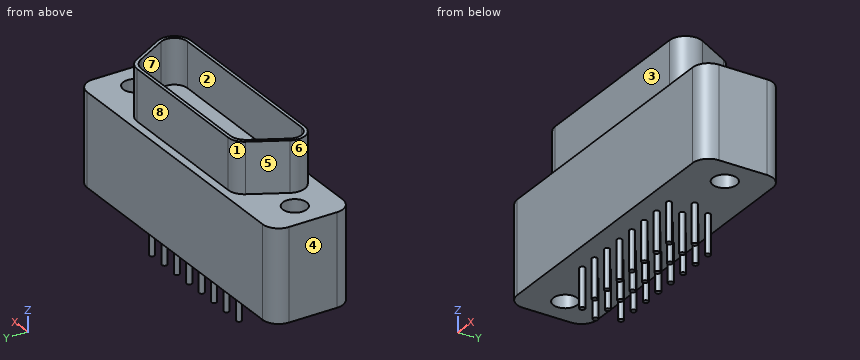
from build123d import *

# Parameters (mm, degrees)
F0_R     = 1.1684
F1_DEPTH = 4.5085
F3_DEPTH = 4.953
F5_DEPTH = 4.4069
F6_R     = 0.254
F7_DEPTH = 3.81


with BuildPart() as f1:
    # F0 (on Top) → F1 (new body, symmetric)
    with BuildSketch(Plane.XY):
        with BuildLine():
            Line((13.4747, 3.937), (-13.4747, 3.937))
            ThreePointArc((-13.4747, 3.937), (-14.588252, 3.475752), (-15.0495, 2.3622))
            Line((-15.0495, 2.3622), (-15.0495, -2.3622))
            ThreePointArc((-15.0495, -2.3622), (-14.588252, -3.475752), (-13.4747, -3.937))
            Line((-13.4747, -3.937), (13.4747, -3.937))
            ThreePointArc((13.4747, -3.937), (14.588252, -3.475752), (15.0495, -2.3622))
            Line((15.0495, -2.3622), (15.0495, 2.3622))
            ThreePointArc((15.0495, 2.3622), (14.588252, 3.475752), (13.4747, 3.937))
        make_face()
        with Locations((-12.2555, 0)):
            Circle(F0_R, mode=Mode.SUBTRACT)
        with Locations((12.2555, 0)):
            Circle(F0_R, mode=Mode.SUBTRACT)
    extrude(amount=F1_DEPTH, both=True)

    # F2 (on face) → F3 (join)
    with BuildSketch(Plane.XY.offset(4.5085)):
        with BuildLine():
            Line((-8.78192, -3.2004), (8.783378, -3.2004))
            ThreePointArc((8.783378, -3.2004), (10.140271, -2.424871), (10.160729, -0.862122))
            Line((10.160729, -0.862122), (8.372639, 2.363678))
            ThreePointArc((8.372639, 2.363678), (7.794559, 2.957094), (6.995288, 3.175))
            Line((6.995288, 3.175), (-6.99383, 3.175))
            ThreePointArc((-6.99383, 3.175), (-7.793101, 2.957094), (-8.371181, 2.363678))
            Line((-8.371181, 2.363678), (-10.159271, -0.862122))
            ThreePointArc((-10.159271, -0.862122), (-10.138814, -2.424871), (-8.78192, -3.2004))
        make_face()
    extrude(amount=F3_DEPTH)

    # F4 (on face) → F5 (cut)
    with BuildSketch(Plane.XY.offset(9.4615)):
        with BuildLine():
            Line((6.808266, 2.8575), (-6.806808, 2.8575))
            ThreePointArc((-6.806808, 2.8575), (-7.60608, 2.639594), (-8.184159, 2.046178))
            Line((-8.184159, 2.046178), (-9.871127, -0.997192))
            ThreePointArc((-9.871127, -0.997192), (-9.854629, -2.257474), (-8.76036, -2.8829))
            Line((-8.76036, -2.8829), (8.761817, -2.8829))
            ThreePointArc((8.761817, -2.8829), (9.856086, -2.257474), (9.872584, -0.997192))
            Line((9.872584, -0.997192), (8.185617, 2.046178))
            ThreePointArc((8.185617, 2.046178), (7.607537, 2.639594), (6.808266, 2.8575))
        make_face()
    extrude(amount=-F5_DEPTH, mode=Mode.SUBTRACT)

    # F6 (on face) → F7 (join)
    with BuildSketch(Plane(origin=(0, 0, -4.5085), x_dir=(1, 0, 0), z_dir=(0, 0, -1))):
        with Locations((-6.6548, 1.905)):
            Circle(F6_R)
        with Locations((-4.7498, 1.905)):
            Circle(F6_R)
        with Locations((-2.8448, 1.905)):
            Circle(F6_R)
        with Locations((-0.9398, 1.905)):
            Circle(F6_R)
        with Locations((0.9652, 1.905)):
            Circle(F6_R)
        with Locations((2.8702, 1.905)):
            Circle(F6_R)
        with Locations((4.7752, 1.905)):
            Circle(F6_R)
        with Locations((6.6802, 1.905)):
            Circle(F6_R)
        with Locations((-7.6073, 0)):
            Circle(F6_R)
        with Locations((-5.7023, 0)):
            Circle(F6_R)
        with Locations((-3.7973, 0)):
            Circle(F6_R)
        with Locations((-1.8923, 0)):
            Circle(F6_R)
        with Locations((0.0127, 0)):
            Circle(F6_R)
        with Locations((1.9177, 0)):
            Circle(F6_R)
        with Locations((-6.6548, -1.905)):
            Circle(F6_R)
        with Locations((-4.7498, -1.905)):
            Circle(F6_R)
        with Locations((-2.8448, -1.905)):
            Circle(F6_R)
        with Locations((-0.9398, -1.905)):
            Circle(F6_R)
        with Locations((0.9652, -1.905)):
            Circle(F6_R)
        with Locations((2.8702, -1.905)):
            Circle(F6_R)
        with Locations((3.8227, 0)):
            Circle(F6_R)
        with Locations((5.7277, 0)):
            Circle(F6_R)
        with Locations((7.6327, 0)):
            Circle(F6_R)
        with Locations((4.7752, -1.905)):
            Circle(F6_R)
        with Locations((6.6802, -1.905)):
            Circle(F6_R)
    extrude(amount=F7_DEPTH)


solid = f1.part
Input: part model. Units: mm. Frame: model coordinates. Face numbers are marked on the shaded views. A direction names the side the tool comes from. Coordinates: 2 decimals unless noted, no trailing zeros. Order: outer loops, then holes, each group sorted by start corner. A loop starts at its lowest first (then second) coordinate and runs counter-clockwise, first axis right, second up. Notation, with made-up numbers: M 70.25,-35 L 89.25,-35 A29 cw 89.25,-10 Z; hole C 72,-40 d2. An arc over 180 degrees is marked long. One line per question, with ' | ' between items.
Item 1: Draft query along Y for the marked faces 1, 2, 3 and 4. Return one class per face: released by +Y, released by -Y, zero draft, split by the parting line, or undercut.
Geometry results:
face 1: released by +Y | face 2: undercut | face 3: released by -Y | face 4: zero draft
Item 2: Pin query (flat end, axial travel): pin 1 (4 mm diameter, centred on x = 5, y = -0.5, fed in from +Z); pin 2 (3.5 mm diameter, centred on x = -2, z = 6.5, fed in from -Y); pin 3 (2 mm diameter, centred on x = -12.26, y = 0, fed in from +Z); pin 4 (1 mm diameter, centred on y = 2, z = -6, fed in from -X). Return the tip coordinate at first contact, or that it passes through.
Geometry results:
pin 1: stops at z = 5.05 | pin 2: stops at y = -3.2 | pin 3: passes through | pin 4: stops at x = -6.91
Item 3: Section A-A (x = -12). Output: boundary loops of the cut face in (y, z), then the cut area to 3 significant figures.
Geometry results:
outline: M -3.94,-4.51 L -1.14,-4.51 L -1.14,4.51 L -3.94,4.51 Z; M 1.14,-4.51 L 3.94,-4.51 L 3.94,4.51 L 1.14,4.51 Z | area: 50.4 mm^2
Item 4: Section B-B (z = -5). Give the number of separate pieces and of enclosed holes in the cut face, then the cut area to 3 significant figures.
Geometry results:
separate pieces: 25 | enclosed holes: 0 | area: 5.07 mm^2
Item 5: Reachability of the marked faces 5, 6, 7 and 8 from +Z, -Z, +X, -X, +Y, -Y: full face, straight path, thin tool, end or side. Return the list, or none.
Geometry results:
face 5: +Z, -X, +Y | face 6: +Z, -X | face 7: +Z | face 8: +Z, +X, -X, +Y
Item 6: Ray query, line 1 along X through (y, z) = (-0.5, 4); line 2 along Y through (x, z) = (-4.5, 6.75) (1 decimal); line 3 along X through (y, z) = (-0.75, 1.75). Return the intervals inside material, ascending.
Geometry results:
line 1: x = -15.05 to -13.31, -11.2 to 11.2, 13.31 to 15.05 | line 2: y = -3.2 to -2.9, 2.9 to 3.2 | line 3: x = -15.05 to -13.15, -11.36 to 11.36, 13.15 to 15.05
